Autodesk Inventor part; units mm, degrees
ref_plane "YZ Plane" through (0, 0, 0) normal (1, 0, 0) x (0, 1, 0)
ref_plane "XZ Plane" through (0, 0, 0) normal (0, 1, 0) x (-1, 0, 0)
ref_plane "XY Plane" through (0, 0, 0) normal (0, 0, 1) x (1, 0, 0)
sketch "Sketch1" plane through (0, 0, 0) normal (0, 0, 1) x (1, 0, 0)
  line L0 (-9.2249, 16.9065) -> (-9.2249, 86.9065)
  line L1 (0.7751, 86.9065) -> (0.7751, 16.9065)
  arc A0 (-9.2249, 16.9065) -> (-4.2249, 11.9065) centre (-4.2249, 16.9065) ccw
  arc A1 (-4.2249, 11.9065) -> (0.7751, 16.9065) centre (-4.2249, 16.9065) ccw
  arc A2 (0.7751, 86.9065) -> (-4.2249, 91.9065) centre (-4.2249, 86.9065) ccw
  arc A3 (-4.2249, 91.9065) -> (-9.2249, 86.9065) centre (-4.2249, 86.9065) ccw
  circle A4 centre (-4.2249, 16.9065) radius 2
  line L2 (-4.2249, 11.9065) -> (-4.2249, 91.9065) construction
  line L3 (0.7751, 16.9065) -> (-9.2249, 16.9065) construction
  point P0 (0, 0)
  point P1 (-9.2249, 91.9065)
  point P2 (-9.2249, 11.9065)
  point P3 (0.7751, 91.9065)
  point P4 (-4.2249, 11.9065)
  dimension "d0" = 10
  dimension "d1" = 80
  dimension "d2" = 5
  dimension "d3" = 4
extrude "Extrusion1" add sketch "Sketch1" along normal blind 1.5
sketch "Sketch2" plane through (0, 0, 1.5) normal (0, 0, 1) x (1, 0, 0)
  circle A0 centre (-4.7249, 87.843) radius 2
  line L0 (-9.2249, 86.9065) -> (-9.2249, 16.9065)
  line L1 (0.7751, 16.9065) -> (0.7751, 86.9065)
  line L2 (0.7751, 85.9065) -> (-9.2249, 85.9065) construction
  circle A1 centre (-4.2249, 85.9065) radius 4
  line L3 (-4.2249, 85.9065) -> (-4.2249, 25.9065)
  line L4 (-4.2249, 25.9065) -> (-0.2249, 25.9065)
  line L5 (-0.2249, 25.9065) -> (-0.2249, 85.9065)
  circle A2 centre (-2.2249, 25.9065) radius 2
  arc A3 (0.7751, 86.9065) -> (-9.2249, 86.9065) centre (-4.2249, 86.9065) ccw
  point P0 (0, 0)
  point P1 (-5.2249, 89.7795)
  point P2 (-4.2249, 81.9065)
  point P3 (-4.2249, 91.9065)
  dimension "d6" = 4
  dimension "d8" = 8
  dimension "d7" = 4.5
  dimension "d9" = 4
  dimension "d10" = 60
  dimension "d13" = 6
extrude "Extrusion2" cut sketch "Sketch2" against normal blind 1.5 contours A0 | A0 A1 L3 | A1 L5 A2 L3 | A2 L4 | L4 A2 picked at (-3.9282, 83.2733)
properties part number "držák" material "Aluminum 6061"
Verification items for the finished model (mm, model axes). A direction names the side the tool comes from. Give positions to 0.01 mm unless a question says otherwise; leave off trailing zeros. Write each loop counter-clockwise with the first axis right and the second up, starting at its lowest first coordinate (ties: lowest second). Pieces come first, ordered by that corner, then holes.
(1) Access from +Z, -Z, +X, -X, +Y, -Y to the whole of each face (thin tool, end or side, straight path). Record for faces 5 (the face through (-1.74, 89.04, 0.76)), 6 (the face through (-9.225, 51, 1)).
(2) Cross-section at A-A (y = 31). Enter the section's corners in (x, z), plus the area to 3 significant figures.
(3) Material ranges on line 1 (X direction, y = 69, z = 0.25); line 2 (Y direction, x = -3, z = 0.75); line 3 (Y direction, x = -5.25, z = 0.4), recorded low to high.
(4) Mould release check, pull along Y, two halves, no side actions. Record for faces 1 (the face through (-4.335, 91.905, 0.74)), 2 (the face through (-4.115, 11.908, 0.74)), 3 (the face through (0.775, 52, 1)), 4 (the face through (-6.672, 87.386, 0.76)): +Y half, -Y half, draft (parallel to the pull), parting line (faces both ways), or undercut.
(5) Cross-section at B-B (z = 0.4). Enter the section's corners in (x, y), plus the area to 3 significant figures.
(6) Cross-section at C-C (x = -7.5). Enter the section's corners in (y, z), plus the area to 3 significant figures.
Worked out:
1. face 5: +Z, -Z
1. face 6: +Z, -Z, -X, +Y, -Y
2. outline: (-9.22, 0) - (-4.22, 0) - (-4.22, 1.5) - (-9.22, 1.5) - close; (-0.22, 0) - (0.78, 0) - (0.78, 1.5) - (-0.22, 1.5) - close
2. area: 9.00 mm2
3. line 1: x = -9.22 to -4.22, -0.22 to 0.78
3. line 2: y = 12.06 to 15.33, 18.49 to 24.06, 89.71 to 91.75
3. line 3: y = 12.01 to 15.19, 18.62 to 85.91, 89.77 to 91.8
4. face 1: +Y half
4. face 2: -Y half
4. face 3: draft
4. face 4: undercut
5. outline: (-9.22, 16.91) arc R5 ccw to (0.78, 16.91) - (0.78, 86.91) arc R5 ccw to (-9.22, 86.91) - close; hole circle Ø4 at (-4.22, 16.91); hole (-5.22, 89.78) arc R2 ccw to (-4.22, 85.91) - (-4.22, 25.91) arc R2 ccw to (-0.22, 25.91) - (-0.22, 85.91) arc R4 ccw to start
5. area: 499 mm2
6. outline: (13.13, 0) - (90.68, 0) - (90.68, 1.5) - (13.13, 1.5) - close
6. area: 116 mm2
